Check sheet for the modelled part. Datum: model origin and axes. Units: mm. A direction names the side the tool comes from. Round coordinates to 2 decimals unless told otherwise and drop trailing zeros. Write each loop counter-clockwise with the first axis right and the second up, starting at its lowest first coordinate (ties: lowest second). Pieces come first, ordered by that corner, then holes.
Item 1: Section check D-D, the plane y = 2.5. Record the cut outline in (x, z), plus the area to 3 significant figures.
Item 2: Depth check by flat-ended pin: pin 1 (0.8 mm diameter, centred on y = 7.5, z = 3, fed in from +X); pin 2 (0.5 mm diameter, centred on x = -4.5, y = 7.5, fed in from -Z); pin 3 (1.1 mm diameter, centred on y = 7.5, z = 7.5, fed in from -X). Enter the tip coordinate at first touch or a pass-through.
Item 3: Section check B-B, the plane y = 0.75. Record the cut outline in (x, z), plus the area to 3 significant figures.
Item 4: Release check for a two-part mould opening along X. For faces 1 (the flat face through (8.4, 4, 0)), 2 (the flat face through (-8.4, 4, 0)), 3 (the flat face through (3.9, 7.5, -0.5)), 4 (the flat face through (7.32, 0.49, -10.63)) record: pulls with the +X half, pulls with the -X half, needs draft (parallel to the pull), parting line crosses it, or undercut.
Item 5: Material ranges on line 1 along X through (y, z) = (7.25, 3.75); line 2 along Z through (x, y) = (-1.5, 6.5); line 3 along X through (y, z) = (3.5, 7.5), recorded low to high.
Item 6: Set-up check for faces 5 (the flat face through (-4, 7.5, 0.5)), 6 (the flat face through (-7.32, 0.49, 10.63)), 7 (the flat face through (0, 7, 0)): record each of +Z, -Z, +X, -X, +Y, -Y from which the full face is reachable in a straight line by a thin tool's end or side.
Item 7: Section check C-C, the plane x = -5.5. Record the cut outline in (y, z).
Item 8: Section check A-A, the plane z = -3.25. Record the cut outline in (x, y), plus the area to 3 significant figures.
from build123d import *

# Parameters (mm, degrees)
SKETCH1_W           = 16.8
SKETCH1_H           = 20.2
SKETCH1_W_2         = 6.9
SKETCH1_H_2         = 3.8
BOSS_EXTRUDE1_DEPTH = 1
SKETCH2_W           = 16.8
SKETCH2_H           = 20.2
SKETCH2_W_2         = 6.9
SKETCH2_H_2         = 3.8
BOSS_EXTRUDE2_DEPTH = 1
SKETCH4_W           = 16.8
SKETCH4_H           = 20.2
SKETCH4_W_2         = 14.8
SKETCH4_H_2         = 18.2
BOSS_EXTRUDE3_DEPTH = 6
SKETCH5_R           = 0.5
BOSS_EXTRUDE4_DEPTH = 1


with BuildPart() as part:
    # Sketch1 → Boss-Extrude1 (new body)
    # profile 1 of 9: a face of its own
    with BuildSketch(Plane(origin=(0, 0, 0), x_dir=(1, 0, 0), z_dir=(0, 1, 0))):
        Rectangle(SKETCH1_W, SKETCH1_H)
        with Locations((3.95, 7.2)):
            Rectangle(SKETCH1_W_2, SKETCH1_H_2, mode=Mode.SUBTRACT)
        with Locations((3.95, 2.4)):
            Rectangle(SKETCH1_W_2, SKETCH1_H_2, mode=Mode.SUBTRACT)
        with Locations((-3.95, -2.4)):
            Rectangle(SKETCH1_W_2, SKETCH1_H_2, mode=Mode.SUBTRACT)
        with Locations((-3.95, -7.2)):
            Rectangle(SKETCH1_W_2, SKETCH1_H_2, mode=Mode.SUBTRACT)
        with Locations((3.95, -7.2)):
            Rectangle(SKETCH1_W_2, SKETCH1_H_2, mode=Mode.SUBTRACT)
        with Locations((3.95, -2.4)):
            Rectangle(SKETCH1_W_2, SKETCH1_H_2, mode=Mode.SUBTRACT)
        with Locations((-3.95, 7.2)):
            Rectangle(SKETCH1_W_2, SKETCH1_H_2, mode=Mode.SUBTRACT)
        with Locations((-3.95, 2.4)):
            Rectangle(SKETCH1_W_2, SKETCH1_H_2, mode=Mode.SUBTRACT)
    # profile 2 of 9: a face of its own
    with BuildSketch(Plane(origin=(0, 0, 0), x_dir=(1, 0, 0), z_dir=(0, 1, 0))):
        with Locations((-3.95, 2.4)):
            Rectangle(SKETCH1_W_2, SKETCH1_H_2)
    # profile 3 of 9: a face of its own
    with BuildSketch(Plane(origin=(0, 0, 0), x_dir=(1, 0, 0), z_dir=(0, 1, 0))):
        with Locations((-3.95, 7.2)):
            Rectangle(SKETCH1_W_2, SKETCH1_H_2)
    # profile 4 of 9: a face of its own
    with BuildSketch(Plane(origin=(0, 0, 0), x_dir=(1, 0, 0), z_dir=(0, 1, 0))):
        with Locations((3.95, 7.2)):
            Rectangle(SKETCH1_W_2, SKETCH1_H_2)
    # profile 5 of 9: a face of its own
    with BuildSketch(Plane(origin=(0, 0, 0), x_dir=(1, 0, 0), z_dir=(0, 1, 0))):
        with Locations((3.95, 2.4)):
            Rectangle(SKETCH1_W_2, SKETCH1_H_2)
    # profile 6 of 9: a face of its own
    with BuildSketch(Plane(origin=(0, 0, 0), x_dir=(1, 0, 0), z_dir=(0, 1, 0))):
        with Locations((3.95, -2.4)):
            Rectangle(SKETCH1_W_2, SKETCH1_H_2)
    # profile 7 of 9: a face of its own
    with BuildSketch(Plane(origin=(0, 0, 0), x_dir=(1, 0, 0), z_dir=(0, 1, 0))):
        with Locations((-3.95, -2.4)):
            Rectangle(SKETCH1_W_2, SKETCH1_H_2)
    # profile 8 of 9: a face of its own
    with BuildSketch(Plane(origin=(0, 0, 0), x_dir=(1, 0, 0), z_dir=(0, 1, 0))):
        with Locations((-3.95, -7.2)):
            Rectangle(SKETCH1_W_2, SKETCH1_H_2)
    # profile 9 of 9: a face of its own
    with BuildSketch(Plane(origin=(0, 0, 0), x_dir=(1, 0, 0), z_dir=(0, 1, 0))):
        with Locations((3.95, -7.2)):
            Rectangle(SKETCH1_W_2, SKETCH1_H_2)
    extrude(amount=BOSS_EXTRUDE1_DEPTH)



with BuildPart() as body_2:
    # Sketch2 → Boss-Extrude2 (new body)
    with BuildSketch(Plane(origin=(0, 7, 0), x_dir=(1, 0, 0), z_dir=(0, 1, 0))):
        Rectangle(SKETCH2_W, SKETCH2_H)
        with Locations((-3.95, -7.2)):
            Rectangle(SKETCH2_W_2, SKETCH2_H_2, mode=Mode.SUBTRACT)
        with Locations((3.95, -7.2)):
            Rectangle(SKETCH2_W_2, SKETCH2_H_2, mode=Mode.SUBTRACT)
        with Locations((3.95, -2.4)):
            Rectangle(SKETCH2_W_2, SKETCH2_H_2, mode=Mode.SUBTRACT)
        with Locations((-3.95, -2.4)):
            Rectangle(SKETCH2_W_2, SKETCH2_H_2, mode=Mode.SUBTRACT)
        with Locations((-3.95, 2.4)):
            Rectangle(SKETCH2_W_2, SKETCH2_H_2, mode=Mode.SUBTRACT)
        with Locations((3.95, 2.4)):
            Rectangle(SKETCH2_W_2, SKETCH2_H_2, mode=Mode.SUBTRACT)
        with Locations((3.95, 7.2)):
            Rectangle(SKETCH2_W_2, SKETCH2_H_2, mode=Mode.SUBTRACT)
        with Locations((-3.95, 7.2)):
            Rectangle(SKETCH2_W_2, SKETCH2_H_2, mode=Mode.SUBTRACT)
    extrude(amount=BOSS_EXTRUDE2_DEPTH)


with BuildPart() as part_1:
    add(part.part)

    add(body_2.part)  # Boss-Extrude3 merges body 2
    # Sketch4 → Boss-Extrude3 (add)
    with BuildSketch(Plane(origin=(0, 1, 0), x_dir=(1, 0, 0), z_dir=(0, 1, 0))):
        Rectangle(SKETCH4_W, SKETCH4_H)
        Rectangle(SKETCH4_W_2, SKETCH4_H_2, mode=Mode.SUBTRACT)
    extrude(amount=BOSS_EXTRUDE3_DEPTH)

    # Sketch5 → Boss-Extrude4 (add)
    # profile 1 of 4: a face of its own
    with BuildSketch(Plane.XZ):
        with BuildLine():
            Line((8.4, 7.47345081), (9.654981825, 10.198339912))
            ThreePointArc((9.654981825, 10.198339912), (9.526374462, 10.99287922), (8.741993026, 11.173373894))
            Line((8.741993026, 11.173373894), (5.940588292, 10.1))
            Line((5.940588292, 10.1), (8.4, 10.1))
            Line((8.4, 10.1), (8.4, 7.47345081))
        make_face()
        with Locations(Location((9, 10.5, 0), (0, 0, 270))):
            Circle(SKETCH5_R, mode=Mode.SUBTRACT)
    # profile 2 of 4: a face of its own
    with BuildSketch(Plane.XZ):
        with BuildLine():
            Line((9.654981825, -10.198339912), (8.4, -7.47345081))
            Line((8.4, -7.47345081), (8.4, -10.1))
            Line((8.4, -10.1), (5.940588292, -10.1))
            Line((5.940588292, -10.1), (8.741993026, -11.173373894))
            ThreePointArc((8.741993026, -11.173373894), (9.526374462, -10.99287922), (9.654981825, -10.198339912))
        make_face()
        with Locations(Location((9, -10.5, 0), (0, 0, 270))):
            Circle(SKETCH5_R, mode=Mode.SUBTRACT)
    # profile 3 of 4: a face of its own
    with BuildSketch(Plane.XZ):
        with BuildLine():
            Line((-8.4, 10.1), (-5.940588292, 10.1))
            Line((-5.940588292, 10.1), (-8.741993026, 11.173373894))
            ThreePointArc((-8.741993026, 11.173373894), (-9.526374462, 10.99287922), (-9.654981825, 10.198339912))
            Line((-9.654981825, 10.198339912), (-8.4, 7.47345081))
            Line((-8.4, 7.47345081), (-8.4, 10.1))
        make_face()
        with Locations(Location((-9, 10.5, 0), (0, 0, 270))):
            Circle(SKETCH5_R, mode=Mode.SUBTRACT)
    # profile 4 of 4: a face of its own
    with BuildSketch(Plane.XZ):
        with BuildLine():
            Line((-8.741993026, -11.173373894), (-5.940588292, -10.1))
            Line((-5.940588292, -10.1), (-8.4, -10.1))
            Line((-8.4, -10.1), (-8.4, -7.47345081))
            Line((-8.4, -7.47345081), (-9.654981825, -10.198339912))
            ThreePointArc((-9.654981825, -10.198339912), (-9.526374462, -10.99287922), (-8.741993026, -11.173373894))
        make_face()
        with Locations(Location((-9, -10.5, 0), (0, 0, 270))):
            Circle(SKETCH5_R, mode=Mode.SUBTRACT)
    extrude(amount=-BOSS_EXTRUDE4_DEPTH)


solid = part_1.part
Values found:
1. outline: (-8.4, -10.1) - (8.4, -10.1) - (8.4, 10.1) - (-8.4, 10.1) - close; hole (-7.4, -9.1) - (7.4, -9.1) - (7.4, 9.1) - (-7.4, 9.1) - close
1. area: 70.0 mm2
2. pin 1: stops at x = 8.4
2. pin 2: stops at z = -10.1
2. pin 3: stops at x = -8.4
3. outline: (-9.65, -10.2) arc R0.72 ccw to (-8.74, -11.17) - (-5.94, -10.1) - (5.94, -10.1) - (8.74, -11.17) arc R0.72 ccw to (9.65, -10.2) - (8.4, -7.47) - (8.4, 7.47) - (9.65, 10.2) arc R0.72 ccw to (8.74, 11.17) - (5.94, 10.1) - (-5.94, 10.1) - (-8.74, 11.17) arc R0.72 ccw to (-9.65, 10.2) - (-8.4, 7.47) - (-8.4, -7.47) - close; hole circle Ø1 at (-9, -10.5); hole circle Ø1 at (-9, 10.5); hole circle Ø1 at (9, -10.5); hole circle Ø1 at (9, 10.5)
3. area: 352 mm2
4. face 1: pulls with the +X half
4. face 2: pulls with the -X half
4. face 3: undercut
4. face 4: undercut
5. line 1: x = -8.4 to -7.4, -0.5 to 0.5, 7.4 to 8.4
5. line 2: z = -10.1 to -9.1, 9.1 to 10.1
5. line 3: x = -8.4 to -7.4, 7.4 to 8.4
6. face 5: +Y
6. face 6: +Z, +Y, -Y
6. face 7: none
7. outline: (0, -10.1) - (8, -10.1) - (8, -9.1) - (1, -9.1) - (1, 9.1) - (8, 9.1) - (8, 10.1) - (0, 10.1) - close; (7, -5.3) - (8, -5.3) - (8, -4.3) - (7, -4.3) - close; (7, -0.5) - (8, -0.5) - (8, 0.5) - (7, 0.5) - close; (7, 4.3) - (8, 4.3) - (8, 5.3) - (7, 5.3) - close
8. outline: (-8.4, 0) - (8.4, 0) - (8.4, 8) - (7.4, 8) - (7.4, 1) - (-7.4, 1) - (-7.4, 8) - (-8.4, 8) - close; (-0.5, 7) - (0.5, 7) - (0.5, 8) - (-0.5, 8) - close
8. area: 31.8 mm2
